from build123d import *

# Parameters (mm, degrees)
F1_DEPTH = 5
F2_R     = 0.5
F3_R     = 0.5
F4_R     = 0.5


with BuildPart() as f1:
    # F0 (on Front) → F1 (new body)
    with BuildSketch(Plane.XZ):
        with BuildLine():
            ThreePointArc((29.600664, 150), (26.215117, 148.679411), (24.617936, 145.415227))
            Line((24.617936, 145.415227), (0.485222, -144.177339))
            ThreePointArc((0.485222, -144.177339), (-1.543199, -148.322853), (-5.842844, -150))
            Line((-5.842844, -150), (-70, -150))
            ThreePointArc((-70, -150), (-73.535534, -151.464466), (-75, -155))
            Line((-75, -155), (-75, -160.025))
            Line((-75, -160.025), (-55, -160.025))
            Line((-55, -160.025), (-55, -164.975))
            Line((-55, -164.975), (-75, -164.975))
            Line((-75, -164.975), (-75, -170))
            ThreePointArc((-75, -170), (-73.535534, -173.535534), (-70, -175))
            Line((-70, -175), (-5.842844, -175))
            ThreePointArc((-5.842844, -175), (15.384539, -166.71991), (25.398866, -146.253476))
            Line((25.398866, -146.253476), (34.674155, -34.95))
            Line((34.674155, -34.95), (25.086655, -34.95))
            Line((25.086655, -34.95), (25.086655, -30))
            Line((25.086655, -30), (35.086655, -30))
            Line((35.086655, -30), (50.041528, 149.458477))
            ThreePointArc((50.041528, 149.458477), (49.911197, 149.838555), (49.543256, 150))
            Line((49.543256, 150), (29.600664, 150))
        make_face()
    extrude(amount=F1_DEPTH)

    # F2
    f2_edges = [f1.edges().sort_by_distance(p)[0] for p in [
        (35.086655, -2.5, -30),
    ]]
    fillet(f2_edges, radius=F2_R)

    # F3
    f3_edges = [f1.edges().sort_by_distance(p)[0] for p in [
        (34.674155, -2.5, -34.95),
    ]]
    fillet(f3_edges, radius=F3_R)

    # F4
    f4_edges = [f1.edges().sort_by_distance(p)[0] for p in [
        (-75, -2.5, -164.975),
        (-75, -2.5, -160.025),
    ]]
    fillet(f4_edges, radius=F4_R)


solid = f1.part
Read the model definition and answer for the solid it produces. Units are mm, in the model's axes. Coordinates: 2 decimals unless noted, no trailing zeros. Order: outer loops, then holes, each group sorted by start corner. A loop starts at its lowest first (then second) coordinate and runs counter-clockwise, first axis right, second up. Notation, with made-up numbers: M -12,52 L 47,52 A15 cw 47,71 Z; hole C 67.5,72.5 d10. An arc over 180 degrees is marked long. Put each result on its own line as item: value. Start each with the question number.
Item 1: Given pin 1 Ø1 at (x, y) = (-25, -1.5) entering from +Z; pin 2 Ø2 at (x, y) = (-2, -4) entering from -Z; pin 3 Ø1.5 at (y, z) = (-1.5, -33.5) entering from +X, each flat-ended and moving along its own axis, determine where each tip first touches the part or whether it passes through.
Item 2: Consider probe 1 along Z at (x, y) = (-52.5, -2.15); probe 2 along X at (y, z) = (-1.6, 10); probe 3 along X at (y, z) = (-3, -16.5) (3 decimals). Determine where each line is inside the solid, lowest interval first. Write a range as [from, to].
Item 3: Section C-C, the plane x = -10.5 is taken. Determine the outline of the cut face in (y, z), plus the area to 3 significant figures.
Item 4: Section A-A, the plane x = -66 is taken. Determine the outline of the cut face in (y, z) (3 decimals).
Item 5: Section B-B, the plane y = -0.85 is taken. Determine the outline of the cut face in (x, z) (3 decimals).
Item 6: Section D-D, the plane z = -61.5 is taken. Determine the outline of the cut face in (x, y) (3 decimals).
Computed:
1. pin 1: stops at z = -150
1. pin 2: stops at z = -174.87
1. pin 3: stops at x = 25.09
2. probe 1: z = [-175, -150]
2. probe 2: x = [13.33, 38.42]
2. probe 3: x = [11.125, 36.212]
3. outline: M -5,-175 L 0,-175 L 0,-150 L -5,-150 Z
3. area: 125 mm2
4. outline: M -5,-175 L 0,-175 L 0,-164.975 L -5,-164.975 Z; M -5,-160.025 L 0,-160.025 L 0,-150 L -5,-150 Z
5. outline: M -75,-170 A5 ccw -70,-175 L -5.843,-175 A31.35 ccw 25.399,-146.253 L 34.629,-35.492 A0.5 ccw 34.131,-34.95 L 25.087,-34.95 L 25.087,-30 L 34.627,-30 A0.5 ccw 35.125,-29.542 L 50.042,149.458 A0.5 ccw 49.543,150 L 29.601,150 A5 ccw 24.618,145.415 L 0.485,-144.177 A6.35 cw -5.843,-150 L -70,-150 A5 ccw -75,-155 L -75,-159.525 A0.5 ccw -74.5,-160.025 L -55,-160.025 L -55,-164.975 L -74.5,-164.975 A0.5 ccw -75,-165.475 Z
6. outline: M 7.375,-5 L 32.462,-5 L 32.462,0 L 7.375,0 Z
